For this review, take the finished solid that the model builds, in its own axes (mm). A direction names the side the tool comes from. Coordinates: 2 decimals unless noted, no trailing zeros. Loops run counter-clockwise (first coordinate to the right, second up) from the corner with the lowest first, then second, coordinate; pieces in that order, holes last. Notation, with made-up numbers: (32.25, -16) - (70.25, -16) arc R14 cw to (70.25, -12) - close; hole circle Ø3 at (19.5, 13). An arc over 180 degrees is marked (long way). One line per item, written item: value. Start each with the question number.
1. Insertion check: pin 1 (3 mm diameter, centred on x = -7, z = 14, fed in from -Y); pin 2 (8 mm diameter, centred on x = -5, y = 8.5, fed in from -Z); pin 3 (1 mm diameter, centred on x = -1, z = 43, fed in from +Y); pin 4 (10 mm diameter, centred on x = 1.5, y = -6.5, fed in from +Z). Each pin has a flat end and moves straight along its axis. Give the tip position at first contact, or say it passes through.
2. Take a section at A-A, the plane x = 5.25. Count the separate pieces of the cut face and the enclosed holes in it, and give its area (3 significant figures).
3. The part is to be moulded in two halves that separate along Z. For faces 1 (the face through (0.14, 25.79, 43.03)), 2 (the face through (0.14, 11.79, 43.03)), 3 (the face through (-12, -32, 58)), 4 (the face through (0, 0, 0)), say which applies: released by +Z, released by -Z, zero draft, split by the parting line, or undercut.
4. Take a section at D-D, the plane z = 41. State the section outline as (x, y) points.
5. Take a section at B-B, the plane z = 47.5. State the section outline as (x, y) points, and give its area (3 significant figures).
6. For faces 5 (the face through (11, 0, 60)), 6 (the face through (0, 0, 44)), list the 3-axis set-ups (+Z, -Z, +X, -X, +Y, -Y) from which the entire face can be reached by the end or side of a thin tool; tool diameter is ignored.
7. To check wall thickness, follow line 1 (Z direction, x = -2.75, y = 14); line 2 (X direction, y = -13, z = 19); line 3 (Y direction, x = 1.5, z = 15). State the ranges of each line that lie inside material, in increasing order. Write a range as from..to.
8. Take a section at C-C, the plane y = 14. State the section outline as (x, z) points.
Autodesk Fusion 360 part; units mm, degrees
sketch "Sketch1" plane through (0, 0, 0) normal (0, 0, 1) x (1, 0, 0)
  line L0 (10, -30) -> (-10, -30)
  line L1 (-10, -33) -> (-10, 33)
  line L2 (-10, 30) -> (10, 30)
  line L3 (10, 33) -> (10, -33)
  line L4 (-13, -33) -> (-13, 33)
  line L5 (-13, 33) -> (13, 33)
  line L6 (13, 33) -> (13, -33)
  line L7 (13, -33) -> (-13, -33)
extrude "Extrude1" add sketch "Sketch1" along normal blind 3
extrude "Extrude2" add sketch "Sketch1" along normal blind 60 contours L3 L5 L6 L7 | L1 L4 L5 L7
sketch "Sketch2" plane through (13, 0, 0) normal (1, 0, 0) x (0, 1, 0)
  line L0 (-33, 0) -> (33, 0)
  line L1 (33, 0) -> (33, 60)
  line L2 (33, 60) -> (-33, 60)
  line L3 (-33, 60) -> (-33, 0)
  circle A0 centre (-28, 55) radius 3
  circle A1 centre (0, 55) radius 3
  circle A2 centre (-14, 55) radius 3
  line L4 (0, 1.75) -> (0, 22.5)
  circle A3 centre (14, 55) radius 3
  circle A4 centre (28, 55) radius 3
  circle A5 centre (-28, 41) radius 3
  circle A6 centre (-14, 41) radius 3
  circle A7 centre (0, 41) radius 3
  circle A8 centre (14, 41) radius 3
  circle A9 centre (28, 41) radius 3
  circle A10 centre (-28, 27) radius 3
  circle A11 centre (-14, 27) radius 3
  circle A12 centre (0, 27) radius 3
  circle A13 centre (14, 27) radius 3
  circle A14 centre (28, 27) radius 3
  circle A15 centre (-28, 13) radius 3
  circle A16 centre (-14, 13) radius 3
  circle A17 centre (0, 13) radius 3
  circle A18 centre (14, 13) radius 3
  circle A19 centre (28, 13) radius 3
  dimension "d8" = 0
  dimension "d9" = -42
extrude "Extrude3" add sketch "Sketch2" against normal blind 26 contours A0 | A1 | A2 | L4 A17 | L4 A17 | A3 | A4 | A5 | A6 | A7 | A8 | A9 | A10 | A11 | A12 | A13 | A14 | A15 | A16 | A18 | A19
fillet "Fillet1" radius 5 4 edges at (11.5, -33, 60) (-11.5, -33, 60) (11.5, 33, 60) (-11.5, 33, 60)
Solutions:
1. pin 1: y = -31
1. pin 2: z = 0
1. pin 3: y = 30.6
1. pin 4: z = 57.6
2. separate pieces: 21
2. enclosed holes: 0
2. area: 763 mm2
3. face 1: undercut
3. face 2: undercut
3. face 3: released by +Z
3. face 4: released by -Z
4. outline: (-13, -33) - (-10, -33) - (-10, -31) - (10, -31) - (10, -33) - (13, -33) - (13, 33) - (10, 33) - (10, 31) - (-10, 31) - (-10, 33) - (-13, 33) - close; hole (-10, -25) - (10, -25) - (10, -17) - (-10, -17) - close; hole (-10, -11) - (10, -11) - (10, -3) - (-10, -3) - close; hole (-10, 3) - (10, 3) - (10, 11) - (-10, 11) - close; hole (-10, 17) - (10, 17) - (10, 25) - (-10, 25) - close
5. outline: (-13, -33) - (-10, -33) - (-10, 33) - (-13, 33) - close; (10, -33) - (13, -33) - (13, 33) - (10, 33) - close
5. area: 396 mm2
6. face 5: +Z, +X, -X, +Y, -Y
6. face 6: none
7. line 1: 0..3, 10..16, 24..30, 38..44, 52..58
7. line 2: -13..-10, 10..13
7. line 3: -30.24..-25.76, -16.24..-11.76, -2.24..2.24, 11.76..16.24, 25.76..30.24
8. outline: (-13, 0) - (13, 0) - (13, 60) - (10, 60) - (10, 58) - (-10, 58) - (-10, 60) - (-13, 60) - close; hole (-10, 3) - (10, 3) - (10, 10) - (-10, 10) - close; hole (-10, 16) - (10, 16) - (10, 24) - (-10, 24) - close; hole (-10, 30) - (10, 30) - (10, 38) - (-10, 38) - close; hole (-10, 44) - (10, 44) - (10, 52) - (-10, 52) - close
